Can you work these out from the model? Positions are in its coordinate system, mm. A direction names the side the tool comes from. Round coordinates to 2 decimals unless told otherwise and drop trailing zeros. Loops run counter-clockwise (first coordinate to the right, second up) from the corner with the lowest first, then second, coordinate; pieces in that order, holes last. Notation, with made-up numbers: (13.25, 88.5) -> (20.25, 88.5) arc R25 ccw to (20.25, 120.5) -> close; hole circle Ø8 at (40.5, 79). An arc over 180 degrees is marked (long way). Write each question's results on one line, items separated by ' | '.
from build123d import *

# Parameters (mm, degrees)
SKETCH1_W           = 85
SKETCH1_H           = 77
BOSS_EXTRUDE1_DEPTH = 1.25
SKETCH3_R           = 17.907
SKETCH3_R_2         = 13.97
BOSS_EXTRUDE3_DEPTH = 4.7625
BOSS_EXTRUDE7_DEPTH = 26
SKETCH6_W           = 77
SKETCH6_H           = 2.5
BOSS_EXTRUDE8_DEPTH = 2.5


with BuildPart() as part:
    # Sketch1 → Boss-Extrude1 (new body)
    with BuildSketch(Plane(origin=(0, 0, 0), x_dir=(1, 0, 0), z_dir=(0, 1, 0))):
        Rectangle(SKETCH1_W, SKETCH1_H)
    extrude(amount=BOSS_EXTRUDE1_DEPTH)

    # Sketch3 → Boss-Extrude3 (add)
    # profile 1 of 2: a face of its own
    with BuildSketch(Plane(origin=(0, 1.25, 0), x_dir=(1, 0, 0), z_dir=(0, 1, 0))):
        with Locations(Location((19.133331774, 0, 0), (0, 0, 90))):
            Circle(SKETCH3_R)
        with Locations(Location((19.133331774, 0, 0), (0, 0, 90))):
            Circle(SKETCH3_R_2, mode=Mode.SUBTRACT)
    # profile 2 of 2: a face of its own
    with BuildSketch(Plane(origin=(0, 1.25, 0), x_dir=(1, 0, 0), z_dir=(0, 1, 0))):
        with Locations(Location((-19.133331774, 0, 0), (0, 0, 90))):
            Circle(SKETCH3_R)
        with Locations(Location((-19.133331774, 0, 0), (0, 0, 90))):
            Circle(SKETCH3_R_2, mode=Mode.SUBTRACT)
    extrude(amount=BOSS_EXTRUDE3_DEPTH)

    # Sketch4 → Boss-Extrude7 (add)
    with BuildSketch(Plane(origin=(0, 1.25, 0), x_dir=(1, 0, 0), z_dir=(0, 1, 0))):
        with BuildLine():
            ThreePointArc((-34.668002675, 8.907), (-31.887785522, 12.569190849), (-28.266663548, 15.402691314))
            Line((-28.266663548, 15.402691314), (-28.266663548, 17.907))
            Line((-28.266663548, 17.907), (-38.266663548, 17.907))
            Line((-38.266663548, 17.907), (-38.266663548, 8.907))
            Line((-38.266663548, 8.907), (-34.668002675, 8.907))
        make_face()
        with BuildLine():
            ThreePointArc((-28.266663548, -15.402691314), (-31.887785522, -12.569190849), (-34.668002675, -8.907))
            Line((-34.668002675, -8.907), (-38.266663548, -8.907))
            Line((-38.266663548, -8.907), (-38.266663548, -17.907))
            Line((-38.266663548, -17.907), (-28.266663548, -17.907))
            Line((-28.266663548, -17.907), (-28.266663548, -15.402691314))
        make_face()
        with BuildLine():
            Line((0, -8.907), (-3.598660873, -8.907))
            ThreePointArc((-3.598660873, -8.907), (-6.378878026, -12.569190849), (-10, -15.402691314))
            Line((-10, -15.402691314), (-10, -17.907))
            Line((-10, -17.907), (0, -17.907))
            Line((0, -17.907), (0, -8.907))
        make_face()
        with BuildLine():
            ThreePointArc((10, -15.402691314), (6.378878026, -12.569190849), (3.598660873, -8.907))
            Line((3.598660873, -8.907), (0, -8.907))
            Line((0, -8.907), (0, -17.907))
            Line((0, -17.907), (10, -17.907))
            Line((10, -17.907), (10, -15.402691314))
        make_face()
        with BuildLine():
            Line((0, 8.907), (0, 17.907))
            Line((0, 17.907), (-10, 17.907))
            Line((-10, 17.907), (-10, 15.402691314))
            ThreePointArc((-10, 15.402691314), (-6.378878026, 12.569190849), (-3.598660873, 8.907))
            Line((-3.598660873, 8.907), (0, 8.907))
        make_face()
        with BuildLine():
            Line((10, 17.907), (0, 17.907))
            Line((0, 17.907), (0, 8.907))
            Line((0, 8.907), (3.598660873, 8.907))
            ThreePointArc((3.598660873, 8.907), (6.378878026, 12.569190849), (10, 15.402691314))
            Line((10, 15.402691314), (10, 17.907))
        make_face()
        with BuildLine():
            Line((28.266663548, 17.907), (28.266663548, 15.402691314))
            ThreePointArc((28.266663548, 15.402691314), (31.887785522, 12.569190849), (34.668002675, 8.907))
            Line((34.668002675, 8.907), (38.266663548, 8.907))
            Line((38.266663548, 8.907), (38.266663548, 17.907))
            Line((38.266663548, 17.907), (28.266663548, 17.907))
        make_face()
        with BuildLine():
            ThreePointArc((34.668002675, -8.907), (31.887785522, -12.569190849), (28.266663548, -15.402691314))
            Line((28.266663548, -15.402691314), (28.266663548, -17.907))
            Line((28.266663548, -17.907), (38.266663548, -17.907))
            Line((38.266663548, -17.907), (38.266663548, -8.907))
            Line((38.266663548, -8.907), (34.668002675, -8.907))
        make_face()
    extrude(amount=BOSS_EXTRUDE7_DEPTH)

    # Sketch6 → Boss-Extrude8 (add)
    with BuildSketch(Plane.ZY.offset(42.5)):
        Rectangle(SKETCH6_W, SKETCH6_H)
    boss_extrude8 = extrude(amount=BOSS_EXTRUDE8_DEPTH)

    # Mirror1: Boss-Extrude8 across plane
    add(boss_extrude8.mirror(Plane(origin=(0, 0, 0), x_dir=(0, 0, 1), z_dir=(1, 0, 0))))


solid = part.part
1. We'd pull the mould along X, two halves only. Please class faces 4 (the face through (33, 14, -17.907)), 5 (the face through (38.267, 14, 13)), 6 (the face through (-5.496, 3.598, 3.028)): pulls with the +X half, pulls with the -X half, needs draft (parallel to the pull), parting line crosses it, or undercut.
Final values:
face 4: needs draft | face 5: pulls with the +X half | face 6: undercut
2. If we section it at B-B (z = 19): List the corners of the cut face in (x, y) for me.
Final values:
outline: (-45, -1.25) -> (-42.5, -1.25) -> (-42.5, 0) -> (42.5, 0) -> (42.5, -1.25) -> (45, -1.25) -> (45, 1.25) -> (-45, 1.25) -> close
3. Will these pins go through, and if not, where does the flat tip stop? pin 1 (12 mm diameter, centred on y = 13, z = -24.5, fed in from +X); pin 2 (3 mm diameter, centred on y = 10.5, z = -17, fed in from -X); pin 3 (3 mm diameter, centred on x = -36, y = 20.5, fed in from -Z); pin 4 (3 mm diameter, centred on y = 8.5, z = 16.5, fed in from +X).
Final values:
pin 1: through | pin 2: x = -38.27 | pin 3: z = -17.91 | pin 4: x = 38.27
4. If we section it at A-A (y = 12): State how many separate pieces and enclosed holes the cut face has, then the cut area to 3 significant figures.
Final values:
separate pieces: 6 | enclosed holes: 0 | area: 525 mm2
5. On a 3-axis mill with a long thin cutter (end or side, diameter ignored), from which of +Z, -Z, +X, -X, +Y, -Y can I reach the whole of each face in a straight line? I mean faces 1 (the face through (6.33, 16.48, -12.52)), 2 (the face through (-1, 0, -1)), 3 (the face through (-34, 27.25, 14)). Say none if no direction works.
Final values:
face 1: +Y | face 2: +Z, -Z, -Y | face 3: +Z, -Z, +X, -X, +Y
6. Please list where these lines run through material, in increasing order: line 1 (X direction, y = 2.35, z = 0); line 2 (X direction, y = 6.75, z = -14.5); line 3 (X direction, y = 22.25, z = -13). Write a range as from..to.
Final values:
line 1: -37.04..-33.1, -5.16..-1.23, 1.23..5.16, 33.1..37.04 | line 2: -38.27..-29.64, -8.63..8.63, 29.64..38.27 | line 3: -38.27..-31.45, -6.82..6.82, 31.45..38.27
7. If we section it at D-D (x = 25): List the corners of the cut face in (y, z) for me.
Final values:
outline: (0, -38.5) -> (1.25, -38.5) -> (1.25, -16.92) -> (6.01, -16.92) -> (6.01, -12.68) -> (1.25, -12.68) -> (1.25, 12.68) -> (6.01, 12.68) -> (6.01, 16.92) -> (1.25, 16.92) -> (1.25, 38.5) -> (0, 38.5) -> close
8. If we section it at C-C (x = -18): List the corners of the cut face in (y, z) for me.
Final values:
outline: (0, -38.5) -> (1.25, -38.5) -> (1.25, -17.87) -> (6.01, -17.87) -> (6.01, -13.92) -> (1.25, -13.92) -> (1.25, 13.92) -> (6.01, 13.92) -> (6.01, 17.87) -> (1.25, 17.87) -> (1.25, 38.5) -> (0, 38.5) -> close
